from build123d import *

# Parameters (mm, degrees)
SKETCH1_W           = 125
SKETCH1_H           = 103
BOSS_EXTRUDE1_DEPTH = 3
SKETCH2_W           = 4
SKETCH2_H           = 15
BOSS_EXTRUDE2_DEPTH = 3


with BuildPart() as part:
    # Sketch1 → Boss-Extrude1 (new body)
    with BuildSketch(Plane.XY):
        with Locations((-62.5, 51.5)):
            Rectangle(SKETCH1_W, SKETCH1_H)
        Polygon((-15, 93), (-110, 93), (-115, 88), (-115, 56.5), (-110, 51.5), (-15, 51.5), (-10, 56.5), (-10, 88), align=None, mode=Mode.SUBTRACT)
    extrude(amount=BOSS_EXTRUDE1_DEPTH)

    # Sketch2 → Boss-Extrude2 (add)
    with BuildSketch(Plane.XY.offset(3)):
        with Locations((2, 82.5)):
            Rectangle(SKETCH2_W, SKETCH2_H)
        with Locations((2, 22.5)):
            Rectangle(SKETCH2_W, SKETCH2_H)
        with Locations((-127, 22.5)):
            Rectangle(SKETCH2_W, SKETCH2_H)
        with Locations((2, 52.5)):
            Rectangle(SKETCH2_W, SKETCH2_H)
        with Locations((-127, 52.5)):
            Rectangle(SKETCH2_W, SKETCH2_H)
        with Locations((-127, 82.5)):
            Rectangle(SKETCH2_W, SKETCH2_H)
    extrude(amount=-BOSS_EXTRUDE2_DEPTH)


solid = part.part
Can you work these out from the model? Positions are in its coordinate system, mm. A direction names the side the tool comes from. Coordinates: 2 decimals unless noted, no trailing zeros. Order: outer loops, then holes, each group sorted by start corner. A loop starts at its lowest first (then second) coordinate and runs counter-clockwise, first axis right, second up. Notation, with made-up numbers: (24, -1.75) - (33, -1.75) arc R21 ccw to (33, 30.25) - close; hole circle Ø2 at (-15.5, -18). An arc over 180 degrees is marked (long way). Answer as a JSON object with one key per item and string values. Group by question number.
Q1. Imagine slicing it at B-B (y = 63.5). Please give me the cut outline in (x, z), and give its area (3 significant figures).
Q2. We'd pull the mould along X, two halves only. Please class faces 6 (the face through (0, 96, 1)), 7 (the face through (-112.5, 54, 1.5)), 8 (the face through (-129, 82, 2)), 9 (the face through (-12, 90, 1)): +X half, -X half, draft (parallel to the pull), parting line (faces both ways), or undercut.
Q3. On a 3-axis mill with a long thin cutter (end or side, diameter ignored), from which of +Z, -Z, +X, -X, +Y, -Y can I reach the whole of each face in a straight line? I mean faces 1 (the face through (-125, 7, 1)), 2 (the face through (-125, 67, 1)), 3 (the face through (2, 90, 2)), 4 (the face through (2, 60, 2)), 5 (the face through (-112, 91, 1)). Say none if no direction works.
Q4. Imagine slicing it at A-A (x = -60). Please give me the cut outline in (y, z), and give its area (4 significant figures).
Q5. I need wall thicknesses on line 1 (X direction, y = 61, z = 0.55); line 2 (X direction, y = 83.5, z = 0.55); line 3 (Y direction, x = -76, z = 2.9). Which ranges of each line are inside material? Lowest first, please. Write a range as from..to.
Q6. Imagine slicing it at C-C (y = 32.5). Please give me the cut outline in (x, z), and give its area (3 significant figures).
Q7. Will these pins go through, and if not, where does the flat tip stop? P1, Ø4, axis at x = -71.5, y = 14, coming from the -Z side; P2, Ø1.5, axis at y = 99.5, z = 1, coming from the +X side; P3, Ø1.5, axis at x = 2.5, z = 2, coming from the +Y side; P4, Ø0.9, axis at x = -127, z = 1, coming from the -Y side.
Determined:
{
 "1": {"outline": "(-125, 0) - (-115, 0) - (-115, 3) - (-125, 3) - close; (-10, 0) - (0, 0) - (0, 3) - (-10, 3) - close", "area": "60.0 mm2"},
 "2": {"face 6": "+X half", "face 7": "undercut", "face 8": "-X half", "face 9": "undercut"},
 "3": {"face 1": "+Z, -Z, -X, -Y", "face 2": "+Z, -Z, -X", "face 3": "+Z, -Z, +X, +Y", "face 4": "+Z, -Z, +X", "face 5": "+Z, -Z"},
 "4": {"outline": "(0, 0) - (51.5, 0) - (51.5, 3) - (0, 3) - close; (93, 0) - (103, 0) - (103, 3) - (93, 3) - close", "area": "184.5 mm2"},
 "5": {"line 1": "x = -125..-115, -10..0", "line 2": "x = -129..-115, -10..4", "line 3": "y = 0..51.5, 93..103"},
 "6": {"outline": "(-125, 0) - (0, 0) - (0, 3) - (-125, 3) - close", "area": "375 mm2"},
 "7": {"P1": "stops at z = 0", "P2": "stops at x = 0", "P3": "stops at y = 90", "P4": "stops at y = 15"}
}
